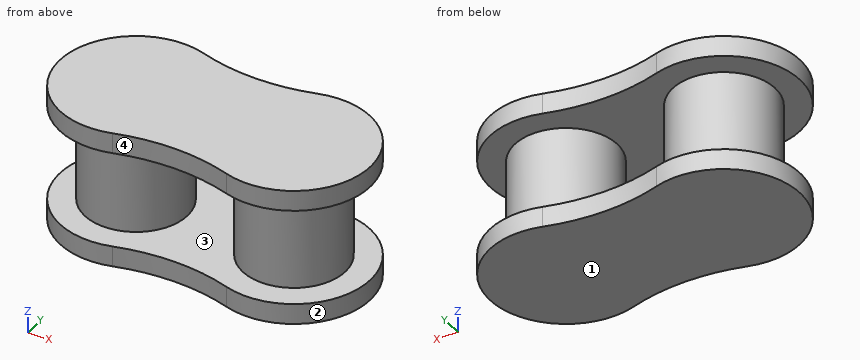
from build123d import *

# Parameters (mm, degrees)
BOSS_EXTRUDE1_DEPTH = 2.032
SKETCH4_R           = 5.08
BOSS_EXTRUDE2_DEPTH = 9.525


with BuildPart() as part:
    # Sketch2 → Boss-Extrude1 (new body)
    with BuildSketch(Plane.XY):
        with BuildLine():
            ThreePointArc((-5.718518673, 7.210065208), (-15.4813, 0), (-5.718518673, -7.210065208))
            ThreePointArc((-5.718518673, -7.210065208), (0, -6.35), (5.718518673, -7.210065208))
            ThreePointArc((5.718518673, -7.210065208), (15.4813, 0), (5.718518673, 7.210065208))
            ThreePointArc((5.718518673, 7.210065208), (0, 6.35), (-5.718518673, 7.210065208))
        make_face()
    boss_extrude1 = extrude(amount=BOSS_EXTRUDE1_DEPTH)

    # Sketch4 → Boss-Extrude2 (add)
    with BuildSketch(Plane.XY.offset(2.032)):
        with Locations(Location((-7.9375, 0, 0), (0, 0, 180))):
            Circle(SKETCH4_R)
        with Locations(Location((7.9375, 0, 0), (0, 0, 180))):
            Circle(SKETCH4_R)
    extrude(amount=BOSS_EXTRUDE2_DEPTH)

    # Mirror1: Boss-Extrude1 across plane
    add(boss_extrude1.mirror(Plane.XY.offset(6.7945)))


solid = part.part
Design review of the part built by this model. Coordinates are the model's own, in mm. Face numbers are marked on the shaded views. A direction names the side the tool comes from. Give positions to 0.01 mm unless a question says otherwise; leave off trailing zeros. Write each loop counter-clockwise with the first axis right and the second up, starting at its lowest first coordinate (ties: lowest second). Pieces come first, ordered by that corner, then holes. Notation, with made-up numbers: M 34.25,44 L 73.25,44 A4 cw 73.25,48 Z; hole C 6.5,54.25 d2. An arc over 180 degrees is marked long. Return JSON: item names as keys, results as strings. Group by question number.
Item 1: Wall thickness on line 1 along Z through (x, y) = (1, 4.75); line 2 along Y through (x, z) = (8, 9); line 3 along X through (y, z) = (-3, 6): over which ranges is each line inside the solid? List them lowest first.
Item 2: The part is to be moulded in two halves that separate along X. For the marked faces 1 and 2, say which applies: pulls with the +X half, pulls with the -X half, needs draft (parallel to the pull), parting line crosses it, or undercut.
Item 3: Take a section at B-B (z = 5.5). Give the boundary of the cut face in (x, y), plus the area to 3 significant figures.
Item 4: Tool access review of the marked faces 3 and 4: name each direction out of +Z, -Z, +X, -X, +Y, -Y from which nothing blocks a thin tool from reaching the whole face with its end or side.
Item 5: Take a section at D-D (y = 0). Give the boundary of the cut face in (x, z), plus the area to 3 significant figures.
Item 6: Take a section at C-C (x = 11). Give the boundary of the cut face in (y, z), plus the area to 3 significant figures.
Item 7: Take a section at A-A (y = -2.5). Give the boundary of the cut face in (x, z) (3 decimals).
Item 8: Clearance check with flat-ended pins moving along their axes: pin 1 Ø1.5 at (y, z) = (3.5, 10.5) entering from -X; pin 2 Ø3 at (y, z) = (-3, 3) entering from -X. State where each tip first meets the part, or that it passes through.
Return value:
{
 "1": {"line 1": "z = 0 to 2.03, 11.56 to 13.59", "line 2": "y = -5.08 to 5.08", "line 3": "x = -12.04 to -3.84, 3.84 to 12.04"},
 "2": {"face 1": "needs draft", "face 2": "undercut"},
 "3": {"outline": "C -7.94,0 d10.16; C 7.94,0 d10.16", "area": "162 mm2"},
 "4": {"face 3": "none", "face 4": "+Z, -Z, -Y"},
 "5": {"outline": "M -15.48,0 L 15.48,0 L 15.48,2.03 L 13.02,2.03 L 13.02,11.56 L 15.48,11.56 L 15.48,13.59 L -15.48,13.59 L -15.48,11.56 L -13.02,11.56 L -13.02,2.03 L -15.48,2.03 Z; hole M -2.86,2.03 L 2.86,2.03 L 2.86,11.56 L -2.86,11.56 Z", "area": "319 mm2"},
 "6": {"outline": "M -6.89,0 L 6.89,0 L 6.89,2.03 L 4.05,2.03 L 4.05,11.56 L 6.89,11.56 L 6.89,13.59 L -6.89,13.59 L -6.89,11.56 L -4.05,11.56 L -4.05,2.03 L -6.89,2.03 Z", "area": "133 mm2"},
 "7": {"outline": "M -15.055,0 L 15.055,0 L 15.055,2.032 L 12.36,2.032 L 12.36,11.557 L 15.055,11.557 L 15.055,13.589 L -15.055,13.589 L -15.055,11.557 L -12.36,11.557 L -12.36,2.032 L -15.055,2.032 Z; hole M -3.515,2.032 L 3.515,2.032 L 3.515,11.557 L -3.515,11.557 Z"},
 "8": {"pin 1": "stops at x = -12.21", "pin 2": "stops at x = -15.25"}
}
